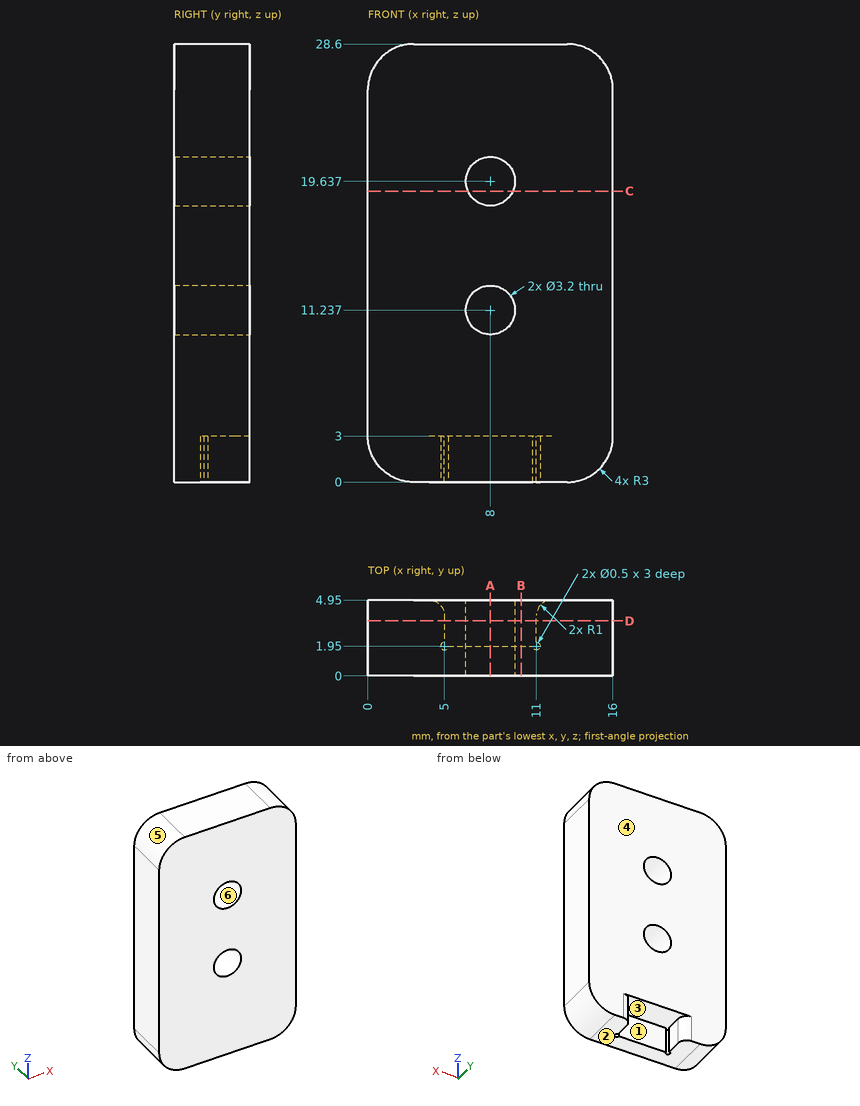
Verification items for this drawing (mm, ordinates from the low corner). A direction names the side the tool comes from. Give positions to 0.01 mm unless a question says otherwise; leave off trailing zeros. Write each loop counter-clockwise with the first axis right and the second up, starting at its lowest first coordinate (ties: lowest second). Pieces come first, ordered by that corner, then holes.
1) Thickness scan on line 1 (Z direction, x = 8, y = 3.4); line 2 (Z direction, x = 6.75, y = 1.7) (1 decimal); line 3 (Z direction, x = 5.5, y = 3.6). Record the ranges inside material, lowest first.
Values follow:
line 1: z = 3 to 9.64, 12.84 to 18.04, 21.24 to 28.6
line 2: z = 0 to 10.2, 12.2 to 18.6, 20.6 to 28.6
line 3: z = 3 to 28.6
2) Cross-section at D-D (y = 3.6). Record the boundary of the cut face in (x, z).
Values follow:
outline: (0, 3) arc R3 ccw to (3, 0) - (5, 0) - (5, 3) - (11, 3) - (11, 0) - (13, 0) arc R3 ccw to (16, 3) - (16, 25.6) arc R3 ccw to (13, 28.6) - (3, 28.6) arc R3 ccw to (0, 25.6) - close; hole circle Ø3.2 at (8, 11.24); hole circle Ø3.2 at (8, 19.64)
3) Cross-section at C-C (z = 19). Record the boundary of the cut face in (x, y).
Values follow:
outline: (0, 0) - (6.53, 0) - (6.53, 4.95) - (0, 4.95) - close; (9.47, 0) - (16, 0) - (16, 4.95) - (9.47, 4.95) - close
4) Release check for a two-part mould opening along Z. For the marked faces 3, 4, 5 and 6 record: released by +Z, released by -Z, zero draft, split by the parting line, or undercut.
Values follow:
face 3: released by -Z
face 4: zero draft
face 5: released by +Z
face 6: undercut
5) Set-up check for the marked faces 1 and 2: record each of +Z, -Z, +X, -X, +Y, -Y from which the full face is reachable in a straight line by a thin tool's end or side.
Values follow:
face 1: -Z, +Y
face 2: -Z, +X, -X, +Y, -Y
6) Cross-section at A-A (x = 8). Record the boundary of the cut face in (y, z), plus the area to 3 significant figures.
Values follow:
outline: (0, 0) - (1.95, 0) - (1.95, 3) - (4.95, 3) - (4.95, 9.64) - (0, 9.64) - close; (0, 12.84) - (4.95, 12.84) - (4.95, 18.04) - (0, 18.04) - close; (0, 21.24) - (4.95, 21.24) - (4.95, 28.6) - (0, 28.6) - close
area: 101 mm2
7) Go/stop test with flat-tipped pins: pin 1 Ø1.9 at (y, z) = (2.5, 1) entering from +X; pin 2 Ø2.5 at (x, z) = (8, 1.5) entering from +Y; pin 3 Ø2.5 at (x, y) = (8.5, 3.5) entering from -Z. Record where each tip stops, or that it passes through.
Values follow:
pin 1: stops at x = 15.81
pin 2: stops at y = 1.95
pin 3: stops at z = 3
8) Cross-section at B-B (x = 10). Record the boundary of the cut face in (y, z), plus the area to 3 significant figures.
Values follow:
outline: (0, 0) - (1.95, 0) - (1.95, 3) - (4.95, 3) - (4.95, 28.6) - (0, 28.6) - close
area: 133 mm2
